Can you work these out from the model? Positions are in its coordinate system, mm. Face numbers are marked on the shaded views. A direction names the side the tool comes from. Give positions to 0.01 mm unless a question says otherwise; leave off trailing zeros. Order: outer loops, then holes, each group sorted by start corner. A loop starts at its lowest first (then second) coordinate and runs counter-clockwise, first axis right, second up. Notation, with made-up numbers: M 84,-36.5 L 89,-36.5 A28 ccw 89,-12.5 Z; hole C 16.25,1 d10. An arc over 180 degrees is marked long. Write each question's results on one line, items separated by ' | '.
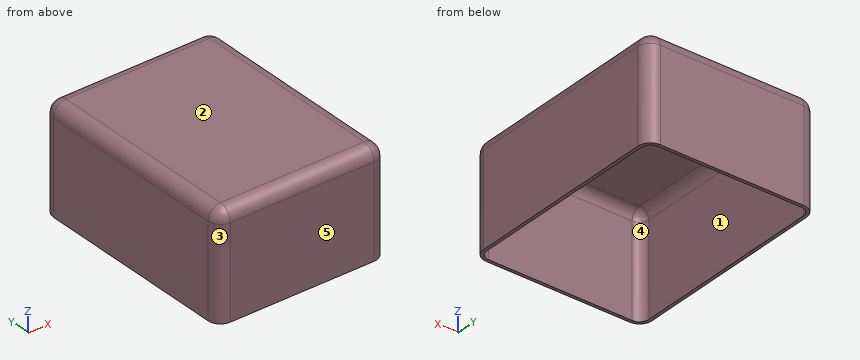
from build123d import *

# Parameters (mm, degrees)
F0_W     = 69.084123
F0_H     = 42.889162
F1_DEPTH = 89.916
F2_R     = 5.08
F3_T     = -1.27


with BuildPart() as f1:
    # F0 (on Front) → F1 (new body)
    with BuildSketch(Plane.XZ):
        with Locations((2.510917, 4.139618)):
            Rectangle(F0_W, F0_H)
    extrude(amount=-F1_DEPTH)

    # F2
    f2_edges = [f1.edges().sort_by_distance(p)[0] for p in [
        (37.052978, 44.958, 25.584199),
        (37.052978, 0, 4.139618),
        (2.510916, 0, 25.584199),
        (-32.031145, 44.958, 25.584199),
        (-32.031145, 0, 4.139618),
        (-32.031145, 89.916, 4.139618),
        (37.052978, 89.916, 4.139618),
        (2.510916, 89.916, 25.584199),
    ]]
    fillet(f2_edges, radius=F2_R)

    # F3
    f3_openings = [f1.faces().sort_by_distance(p)[0] for p in [
        (2.510916, 44.958, -17.304963),
    ]]
    offset(amount=F3_T, openings=f3_openings)


solid = f1.part
(1) Imagine slicing it at A-A, the plane z = -8.5. Write out the boundary of the cut face in (x, y), plus the area to 3 significant figures.
Data:
outline: M -32.03,5.08 A5.08 ccw -26.95,0 L 31.97,0 A5.08 ccw 37.05,5.08 L 37.05,84.84 A5.08 ccw 31.97,89.92 L -26.95,89.92 A5.08 ccw -32.03,84.84 Z; hole M -30.76,5.08 A3.81 ccw -26.95,1.27 L 31.97,1.27 A3.81 ccw 35.78,5.08 L 35.78,84.84 A3.81 ccw 31.97,88.65 L -26.95,88.65 A3.81 ccw -30.76,84.84 Z | area: 388 mm2
(2) Imagine slicing it at C-C, the plane y = 70. Write out the boundary of the cut face in (x, z), plus the area to 3 significant figures.
Data:
outline: M -32.03,-17.3 L -30.76,-17.3 L -30.76,20.5 A3.81 cw -26.95,24.31 L 31.97,24.31 A3.81 cw 35.78,20.5 L 35.78,-17.3 L 37.05,-17.3 L 37.05,20.5 A5.08 ccw 31.97,25.58 L -26.95,25.58 A5.08 ccw -32.03,20.5 Z | area: 189 mm2
(3) For the marked faces 1 and 2, which set-ups out of +Z, -Z, +X, -X, +Y, -Y let a thin tool reach every point of the face, with its end or its side?
Data:
face 1: -Z | face 2: +Z, +X, -X, +Y, -Y
(4) Imagine slicing it at D-D, the plane z = 22. Write out the boundary of the cut face in (x, y), plus the area to 3 significant figures.
Data:
outline: M -31.81,5.08 A4.85 ccw -26.95,0.23 L 31.97,0.23 A4.85 ccw 36.83,5.08 L 36.83,84.84 A4.85 ccw 31.97,89.69 L -26.95,89.69 A4.85 ccw -31.81,84.84 Z; hole M -30.46,5.08 A3.5 ccw -26.95,1.58 L 31.97,1.58 A3.5 ccw 35.48,5.08 L 35.48,84.84 A3.5 ccw 31.97,88.34 L -26.95,88.34 A3.5 ccw -30.46,84.84 Z | area: 410 mm2
(5) We'd pull the mould along X, two halves only. Please class the marked faces 3, 4 and 5: +X half, -X half, draft (parallel to the pull), parting line (faces both ways), or undercut.
Data:
face 3: -X half | face 4: undercut | face 5: draft
(6) Imagine slicing it at B-B, the plane x = -5.5. Write out the boundary of the cut face in (y, z).
Data:
outline: M 0,-17.3 L 1.27,-17.3 L 1.27,20.5 A3.81 cw 5.08,24.31 L 84.84,24.31 A3.81 cw 88.65,20.5 L 88.65,-17.3 L 89.92,-17.3 L 89.92,20.5 A5.08 ccw 84.84,25.58 L 5.08,25.58 A5.08 ccw 0,20.5 Z
(7) Will these pins go through, and if not, where does the flat tip stop? P1, Ø8, axis at x = -25, y = 72.5, coming from the -Z side; P2, Ø1.5, axis at x = -8.5, y = 20, coming from the -Z side.
Data:
P1: stops at z = 23.72 | P2: stops at z = 24.31
(8) I need wall thicknesses on L1, parallel to Y at x = -13, z = -8; L2, parallel to X at y = 70.5, z = -3; L3, parallel to Z at x = 7.5, y = 29. Which ranges of each line are inside material? Lowest first, please. Write a range as from..to.
Data:
L1: y = 0..1.27, 88.65..89.92 | L2: x = -32.03..-30.76, 35.78..37.05 | L3: z = 24.31..25.58
